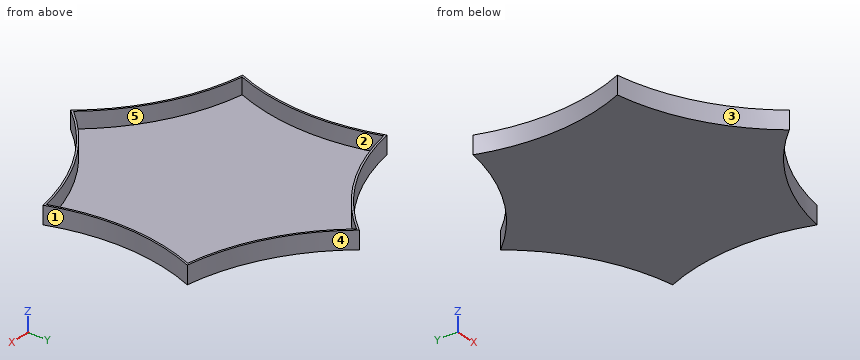
```python
from build123d import *

# Parameters (mm, degrees)
F1_DEPTH = 25
F2_T     = -2.5


with BuildPart() as f1:
    # F0 (on Top) → F1 (new body)
    with BuildSketch(Plane.XY):
        with BuildLine():
            ThreePointArc((-173.205081, 100), (-154.860158, 0), (-173.205081, -100))
            ThreePointArc((-173.205081, -100), (-77.430079, -134.112831), (0, -200))
            ThreePointArc((0, -200), (77.430079, -134.112831), (173.205081, -100))
            ThreePointArc((173.205081, -100), (154.860158, 0), (173.205081, 100))
            ThreePointArc((173.205081, 100), (77.430079, 134.112831), (0, 200))
            ThreePointArc((0, 200), (-77.430079, 134.112831), (-173.205081, 100))
        make_face()
    extrude(amount=F1_DEPTH)

    # F2
    f2_openings = [f1.faces().sort_by_distance(p)[0] for p in [
        (0, 0, 25),
    ]]
    offset(amount=F2_T, openings=f2_openings)


solid = f1.part
```
Here's how the part is built. I have some questions about the finished solid (model axes, mm). Face numbers are marked on the shaded views. A direction names the side the tool comes from. Give positions to 0.01 mm unless a question says otherwise; leave off trailing zeros. Order: outer loops, then holes, each group sorted by start corner. A loop starts at its lowest first (then second) coordinate and runs counter-clockwise, first axis right, second up. Notation, with made-up numbers: (-11, -0.75) -> (36, -0.75) arc R10 ccw to (36, 16.25) -> close; hole circle Ø8 at (24, 83.5). An arc over 180 degrees is marked (long way). Use CSV: the item, a comma, the result in double quotes. Start each with the question number.
Item 1: If I drill on probe 1 along X at (y, z) = (6.5, 19.25); probe 2 along Z at (x, y) = (87.5, 50.5); probe 3 along X at (y, z) = (-181, 3), over which ranges is the centre line in solid material (lowest first)? Write a range as [from, to].
Item 2: Suppose I cut it at B-B (x = 96). List the corners of the cut face in (y, z) for me, and give its area (3 significant figures).
Item 3: On a 3-axis mill with a long thin cutter (end or side, diameter ignored), from which of +Z, -Z, +X, -X, +Y, -Y can I reach the whole of each face in a straight line? I mean the marked faces 1 and 2. Say none if no direction works.
Item 4: I'm going to push flat-ended pins straight in: P1, Ø5, axis at y = 85.5, z = 19.5, coming from the +X side; P2, Ø1.5, axis at x = 86.5, z = 22, coming from the -Y side; P3, Ø10, axis at x = 53, z = 11, coming from the +Y side. Where does each tip first touch, or does it pass through?
Item 5: Suppose I cut it at A-A (z = 10.5). List the corners of the cut face in (x, y) for me, and give its area (3 significant figures).
Item 6: Suppose I cut it at C-C (y = -77.5). List the corners of the cut face in (x, z) for me, and give its area (3 significant figures).
Item 7: Thinking about a two-plate mould opening in Y: for the marked faces 3, 4 and 5, which applies, pulls with the +Y half, pulls with the -Y half, needs draft (parallel to the pull), parting line crosses it, or undercut?
Answer block:
1,probe 1,"x = [-154.94, -152.43], [152.43, 154.94]"
1,probe 2,"z = [0, 2.5]"
1,probe 3,"x = [-16.99, -13.51], [13.51, 16.99]"
2,outline,"(-124.3, 0) -> (124.3, 0) -> (124.3, 25) -> (121.52, 25) -> (121.52, 2.5) -> (-121.52, 2.5) -> (-121.52, 25) -> (-124.3, 25) -> close"
2,area,"746 mm^2"
3,face 1,"+Z, -Z, +X"
3,face 2,"+Z"
4,P1,"stops at x = 168.96"
4,P2,"stops at y = -129.49"
4,P3,"stops at y = 153.66"
5,outline,"(-173.21, -100) arc R281.73 cw to (0, -200) arc R281.73 cw to (173.21, -100) arc R281.73 cw to (173.21, 100) arc R281.73 cw to (0, 200) arc R281.73 cw to (-173.21, 100) arc R281.73 cw to start; hole (-169.8, -98.04) arc R284.23 cw to (0, -196.07) arc R284.23 cw to (169.8, -98.04) arc R284.23 cw to (169.8, 98.04) arc R284.23 cw to (0, 196.07) arc R284.23 cw to (-169.8, 98.04) arc R284.23 cw to start"
5,area,"3,030 mm^2"
6,outline,"(-165.73, 0) -> (165.73, 0) -> (165.73, 25) -> (163.13, 25) -> (163.13, 2.5) -> (-163.13, 2.5) -> (-163.13, 25) -> (-165.73, 25) -> close"
6,area,"946 mm^2"
7,face 3,"pulls with the -Y half"
7,face 4,"pulls with the +Y half"
7,face 5,"undercut"
